Design review of the part built by this model. Coordinates are the model's own, in mm. Coordinates: 2 decimals unless noted, no trailing zeros. Order: outer loops, then holes, each group sorted by start corner. A loop starts at its lowest first (then second) coordinate and runs counter-clockwise, first axis right, second up. Notation, with made-up numbers: M -1.5,53.25 L 47.5,53.25 A8 cw 47.5,66.25 Z; hole C -13.75,80 d3. An arc over 180 degrees is marked long. Answer in a Markdown table with one row per item.
from build123d import *
from OCP.BRepFilletAPI import BRepFilletAPI_MakeFillet

# Parameters (mm, degrees)
SKETCH_1_W          = 170
SKETCH_1_H          = 168
EXTRUDE_1_DEPTH     = 5
SKETCH_3_R          = 40.2
CUT_EXTRUDE_1_DEPTH = 8
SKETCH_5_R          = 2.55
CUT_EXTRUDE_2_DEPTH = 8
SKETCH_7_OUTSIDE_W  = 219.812
SKETCH_7_OUTSIDE_H  = 217.812
CUT_EXTRUDE_3_DEPTH = 8
CUT_EXTRUDE_4_DEPTH = 8
FILLET_1_R          = 10
FILLET_2_R1         = 3
FILLET_2_R2         = 5
SKETCH_9_R          = 1.55
CUT_EXTRUDE_5_DEPTH = 30


with BuildPart() as part:
    # Sketch 1 → Extrude 1 (new body)
    with BuildSketch(Plane.XY):
        Rectangle(SKETCH_1_W, SKETCH_1_H)
    extrude(amount=EXTRUDE_1_DEPTH)

    # Sketch 3 → Cut-Extrude 1 (cut)
    with BuildSketch(Plane.XY.offset(5)):
        Circle(SKETCH_3_R)
    extrude(amount=-CUT_EXTRUDE_1_DEPTH, mode=Mode.SUBTRACT)

    # Sketch 5 → Cut-Extrude 2 (cut)
    with BuildSketch(Plane.XY.offset(5)):
        with Locations((75, 0)):
            Circle(SKETCH_5_R)
        with Locations((75, -74)):
            Circle(SKETCH_5_R)
        with Locations((75, 74)):
            Circle(SKETCH_5_R)
    cut_extrude_2 = extrude(amount=-CUT_EXTRUDE_2_DEPTH, mode=Mode.SUBTRACT)

    # Mirror 1: Cut-Extrude 2 across plane
    add(cut_extrude_2.mirror(Plane(origin=(0, 0, 0), x_dir=(0, 0, 1), z_dir=(1, 0, 0))), mode=Mode.SUBTRACT)

    # Sketch 7 outside → Cut-Extrude 3 (cut)
    with BuildSketch(Plane.XY.offset(5)):
        Rectangle(SKETCH_7_OUTSIDE_W, SKETCH_7_OUTSIDE_H)
        with BuildLine():
            Line((70.514783337, 82.937719591), (0, 47.551279236))
            Line((0, 47.551279236), (-70.514783337, 82.937719591))
            ThreePointArc((-70.514783337, 82.937719591), (-82.118364328, 81.023452804), (-83.876712925, 69.395223387))
            Line((-83.876712925, 69.395223387), (-57.899389351, 19.318256945))
            Line((-57.899389351, 19.318256945), (-79.333333333, 9.012337223))
            ThreePointArc((-79.333333333, 9.012337223), (-85, 0), (-79.333333333, -9.012337223))
            Line((-79.333333333, -9.012337223), (-57.899389351, -19.318256945))
            Line((-57.899389351, -19.318256945), (-83.876712925, -69.395223387))
            ThreePointArc((-83.876712925, -69.395223387), (-82.118364328, -81.023452804), (-70.514783337, -82.937719591))
            Line((-70.514783337, -82.937719591), (0, -47.551279236))
            Line((0, -47.551279236), (70.514783337, -82.937719591))
            ThreePointArc((70.514783337, -82.937719591), (82.118364328, -81.023452804), (83.876712925, -69.395223387))
            Line((83.876712925, -69.395223387), (57.899389351, -19.318256945))
            Line((57.899389351, -19.318256945), (79.333333333, -9.012337223))
            ThreePointArc((79.333333333, -9.012337223), (85, 0), (79.333333333, 9.012337223))
            Line((79.333333333, 9.012337223), (57.899389351, 19.318256945))
            Line((57.899389351, 19.318256945), (83.876712925, 69.395223387))
            ThreePointArc((83.876712925, 69.395223387), (82.118364328, 81.023452804), (70.514783337, 82.937719591))
        make_face(mode=Mode.SUBTRACT)
    extrude(amount=-CUT_EXTRUDE_3_DEPTH, mode=Mode.SUBTRACT)

    # Sketch 8 → Cut-Extrude 4 (cut)
    with BuildSketch(Plane.XY.offset(5)):
        with BuildLine():
            ThreePointArc((50.348751369, -22.136016704), (39.151003806, -38.628990422), (22.809814375, -50.047101496))
            Line((22.809814375, -50.047101496), (68.825352327, -73.139083236))
            Line((68.825352327, -73.139083236), (74.056283345, -67.837463961))
            Line((74.056283345, -67.837463961), (50.348751369, -22.136016704))
        make_face()
        with BuildLine():
            ThreePointArc((-22.809814375, -50.047101496), (-39.151003806, -38.628990422), (-50.348751369, -22.136016704))
            Line((-50.348751369, -22.136016704), (-74.056283345, -67.837463961))
            Line((-74.056283345, -67.837463961), (-68.825352327, -73.139083236))
            Line((-68.825352327, -73.139083236), (-22.809814375, -50.047101496))
        make_face()
        with BuildLine():
            Line((-68.825352327, 73.139083236), (-74.056283345, 67.837463961))
            Line((-74.056283345, 67.837463961), (-50.348751369, 22.136016704))
            ThreePointArc((-50.348751369, 22.136016704), (-39.151003806, 38.628990422), (-22.809814375, 50.047101496))
            Line((-22.809814375, 50.047101496), (-68.825352327, 73.139083236))
        make_face()
        with BuildLine():
            Line((68.825352327, 73.139083236), (22.809814375, 50.047101496))
            ThreePointArc((22.809814375, 50.047101496), (39.151003806, 38.628990422), (50.348751369, 22.136016704))
            Line((50.348751369, 22.136016704), (74.056283345, 67.837463961))
            Line((74.056283345, 67.837463961), (68.825352327, 73.139083236))
        make_face()
    extrude(amount=-CUT_EXTRUDE_4_DEPTH, mode=Mode.SUBTRACT)

    # Fillet 1
    fillet_1_edges = [part.edges().sort_by_distance(p)[0] for p in [
        (57.899389351, 19.318256945, 2.5),
        (57.899389351, -19.318256945, 2.5),
        (0, -47.551279236, 2.5),
        (-57.899389351, -19.318256945, 2.5),
        (-57.899389351, 19.318256945, 2.5),
        (0, 47.551279236, 2.5),
    ]]
    fillet(fillet_1_edges, radius=FILLET_1_R)

    # Fillet 2: one fillet with a radius per group of edges: ONE call of the kernel's fillet builder (fillet() takes one radius for all edges)
    fillet_2_edges_1 = [part.edges().sort_by_distance(p)[0] for p in [
        (-74.056283345, -67.837463961, 2.5),
        (-68.825352327, -73.139083236, 2.5),
        (68.825352327, -73.139083236, 2.5),
        (74.056283345, -67.837463961, 2.5),
        (-68.825352327, 73.139083236, 2.5),
        (-74.056283345, 67.837463961, 2.5),
        (74.056283345, 67.837463961, 2.5),
        (68.825352327, 73.139083236, 2.5),
    ]]
    fillet_2_edges_2 = [part.edges().sort_by_distance(p)[0] for p in [
        (50.348751369, -22.136016704, 2.5),
        (22.809814375, -50.047101496, 2.5),
        (-22.809814375, -50.047101496, 2.5),
        (-50.348751369, -22.136016704, 2.5),
        (-50.348751369, 22.136016704, 2.5),
        (-22.809814375, 50.047101496, 2.5),
        (22.809814375, 50.047101496, 2.5),
        (50.348751369, 22.136016704, 2.5),
    ]]
    fillet_2 = BRepFilletAPI_MakeFillet(part.part.solid().wrapped)
    for e in fillet_2_edges_1:
        fillet_2.Add(FILLET_2_R1, e.wrapped)
    for e in fillet_2_edges_2:
        fillet_2.Add(FILLET_2_R2, e.wrapped)
    add(Compound.cast(fillet_2.Shape()), mode=Mode.REPLACE)

    # Sketch 9 → Cut-Extrude 5 (cut)
    with BuildSketch(Plane.XY.offset(5)):
        with Locations((0, 46)):
            Circle(SKETCH_9_R)
        with Locations((23, 39.837168574)):
            Circle(SKETCH_9_R)
        with Locations((39.837168574, 23)):
            Circle(SKETCH_9_R)
        with Locations((46, 0)):
            Circle(SKETCH_9_R)
        with Locations((39.837168574, -23)):
            Circle(SKETCH_9_R)
        with Locations((23, -39.837168574)):
            Circle(SKETCH_9_R)
        with Locations((0, -46)):
            Circle(SKETCH_9_R)
        with Locations((-23, -39.837168574)):
            Circle(SKETCH_9_R)
        with Locations((-39.837168574, -23)):
            Circle(SKETCH_9_R)
        with Locations((-46, 0)):
            Circle(SKETCH_9_R)
        with Locations((-39.837168574, 23)):
            Circle(SKETCH_9_R)
        with Locations((-23, 39.837168574)):
            Circle(SKETCH_9_R)
    extrude(amount=-CUT_EXTRUDE_5_DEPTH, mode=Mode.SUBTRACT)


solid = part.part
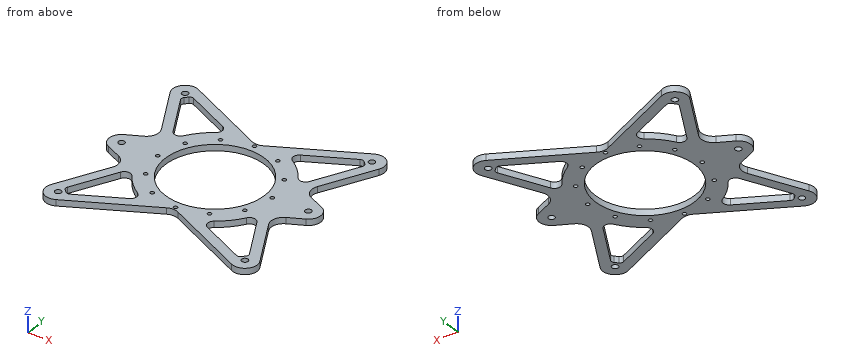
(1) Add section A-A, the plane y = 6.5. Give the boundary of the cut face in (x, z).
Return value:
| item | result |
|---|---|
| outline | M -82.6,0 L -39.67,0 L -39.67,5 L -82.6,5 Z; M 39.67,0 L 82.6,0 L 82.6,5 L 39.67,5 Z |
(2) Add section B-B, the plane x = 9. Give the boundary of the cut face in (y, z).
Return value:
| item | result |
|---|---|
| outline | M -52.07,0 L -39.18,0 L -39.18,5 L -52.07,5 Z; M 39.18,0 L 52.07,0 L 52.07,5 L 39.18,5 Z |
(3) For line 1 along Y through (x, z) = (63.5, 3.95); line 2 along Y through (x, z) = (23, 1.6); line 3 along Y through (x, z) = (-41.5, 0.45), list the stretches that pass through material, from the lowest coordinate up. Write a range as from..to.
Return value:
| item | result |
|---|---|
| line 1 | y = -79.42..-70.47, -47.49..-30.11, -17.89..17.89, 30.11..47.49, 70.47..79.42 |
| line 2 | y = -59.09..-41.39, -38.29..-32.97, 32.97..38.29, 41.39..59.09 |
| line 3 | y = -68.38..-59.43, -36.09..36.09, 59.43..68.38 |
(4) Add section C-C, the plane z = 3.1. Give the number of separate pieces and of enclosed holes in the cut face, and give its area (3 significant figures).
Return value:
| item | result |
|---|---|
| separate pieces | 1 |
| enclosed holes | 23 |
| area | 10,400 mm2 |
